Build history of the part. All positions in model axes, mm. A direction names the side the tool comes from. Coordinates: 2 decimals unless noted, no trailing zeros. Write each loop counter-clockwise with the first axis right and the second up, starting at its lowest first coordinate (ties: lowest second). Pieces come first, ordered by that corner, then holes. Notation, with made-up numbers: M 85.25,16 L 112.25,16 A14 ccw 112.25,33 Z; hole C -5,-4.5 d8. An arc over 180 degrees is marked long. Use CSV: the item, a comma, the result in double quotes. Start each with the question number.
```python
from build123d import *
from OCP.BRepFilletAPI import BRepFilletAPI_MakeChamfer

# Parameters (mm, degrees)
SKETCH_1_R          = 10
EXTRUDE_1_DEPTH     = 16.5
SKETCH_2_R          = 0.5
CUT_EXTRUDE_1_DEPTH = 6
SKETCH_3_R          = 8
CUT_EXTRUDE_2_DEPTH = 0.5
SKETCH_4_R          = 8.75
CUT_EXTRUDE_3_DEPTH = 0.8
SKETCH_5_R          = 0.8
EXTRUDE_2_DEPTH     = 4.85
CHAMFER_1_SIZE      = 2
CHAMFER_1_SIZE2     = 0.2
FILLET_1_R          = 0.4


with BuildPart() as part:
    # Эскиз1 → Бобышка-Вытянуть1 (new body)
    with BuildSketch(Plane.XY):
        Circle(SKETCH_1_R)
    extrude(amount=EXTRUDE_1_DEPTH)

    # Эскиз2 → Вырез-Вытянуть1 (cut)
    with BuildSketch(Plane.XY.offset(16.5)):
        Circle(SKETCH_2_R)
    extrude(amount=-CUT_EXTRUDE_1_DEPTH, mode=Mode.SUBTRACT)

    # Эскиз3 → Вырез-Вытянуть2 (cut)
    with BuildSketch(Plane.XY.offset(16.5)):
        Circle(SKETCH_3_R)
    extrude(amount=-CUT_EXTRUDE_2_DEPTH, mode=Mode.SUBTRACT)

    # Эскиз4 → Вырез-Вытянуть3 (cut)
    with BuildSketch(Plane(origin=(0, 0, 0), x_dir=(-1, 0, 0), z_dir=(0, 0, -1))):
        Circle(SKETCH_4_R)
    extrude(amount=-CUT_EXTRUDE_3_DEPTH, mode=Mode.SUBTRACT)

    # Эскиз5 → Бобышка-Вытянуть2 (add)
    with BuildSketch(Plane(origin=(0, 0, 0.8), x_dir=(-1, 0, 0), z_dir=(0, 0, -1))):
        with Locations((-4.7, 5)):
            Circle(SKETCH_5_R)
        with Locations(Location((4.7, 5, 0), (0, 0, 180))):
            Circle(SKETCH_5_R)
    extrude(amount=EXTRUDE_2_DEPTH)

    # Фаска1: one chamfer whose edges measure the first distance from different faces: ONE call of the kernel's chamfer builder (chamfer() names one face for all edges)
    chamfer_1_edges_1 = [part.edges().sort_by_distance(p)[0] for p in [
        (5.5, 5, -4.05),
    ]]
    chamfer_1_side_1 = [part.faces().sort_by_distance(p)[0] for p in [
        (5.5, 5, -1.625),
    ]]
    chamfer_1_edges_2 = [part.edges().sort_by_distance(p)[0] for p in [
        (-5.5, 5, -4.05),
    ]]
    chamfer_1_side_2 = [part.faces().sort_by_distance(p)[0] for p in [
        (-5.5, 5, -1.625),
    ]]
    chamfer_1 = BRepFilletAPI_MakeChamfer(part.part.solid().wrapped)
    for e in chamfer_1_edges_1:
        chamfer_1.Add(CHAMFER_1_SIZE, CHAMFER_1_SIZE2, e.wrapped, chamfer_1_side_1[0].wrapped)  # the first distance lies on this face
    for e in chamfer_1_edges_2:
        chamfer_1.Add(CHAMFER_1_SIZE, CHAMFER_1_SIZE2, e.wrapped, chamfer_1_side_2[0].wrapped)  # the first distance lies on this face
    add(Compound.cast(chamfer_1.Shape()), mode=Mode.REPLACE)

    # Скругление1
    fillet_1_edges = [part.edges().sort_by_distance(p)[0] for p in [
        (-8, 0, 16.5),
        (-10, 0, 0),
        (8.75, 0, 0),
        (-10, 0, 16.5),
    ]]
    fillet(fillet_1_edges, radius=FILLET_1_R)


solid = part.part
```
1. Slice it at A-A (z = 13.25). List the corners of the cut face in (x, y).
2. Drill centre lines: line 1 along Y through (x, z) = (0, 0.55); line 2 along Y through (x, z) = (0, 13.8); line 3 along Z through (x, y) = (2, 2). Where is each one in solid material? Low to high. Write a range as from..to.
3. Flat gauge pins, fed straight in: pin 1 (1.5 mm diameter, centred on x = -2.5, y = 2, fed in from +Z); pin 2 (2 mm diameter, centred on x = 7, y = 1.5, fed in from +Z); pin 3 (9 mm diameter, centred on x = 0, y = -1, fed in from -Z). Where does each tip first touch, or does it go through?
4. Slice it at C-C (z = -1). List the corners of the cut face in (x, y).
5. Pull direction X, two halves, no side cores. Call faces 1 (the cylindrical face through (5.33, 4.51, -0.61)), 2 (the cylindrical face through (-2.17, -9.76, 8.14)), 3 (the flat face through (-5, 5, -4.05)): pulls with the +X half, pulls with the -X half, needs draft (parallel to the pull), parting line crosses it, or undercut.
6. 3-axis set-ups, long thin cutter, end or side, ignore diameter. For faces 4 (the cylindrical face through (-4.87, 5.78, -0.61)), 5 (the flat face through (0, 0, 10.5)), 6 (the flat face through (5, 5, -4.05)): which of +Z, -Z, +X, -X, +Y, -Y reach the whole face in a straight line?
7. Slice it at B-B (y = 0). List the corners of the cut face in (x, z).
8. Slice it at D-D (z = 7.75). List the corners of the cut face in (x, y), and give its area (3 significant figures).
Established:
1,outline,"C 0,0 d20; hole C 0,0 d1"
2,line 1,"y = -10..-8.75, 8.75..10"
2,line 2,"y = -10..-0.5, 0.5..10"
2,line 3,"z = 0.8..16"
3,pin 1,"stops at z = 16"
3,pin 2,"stops at z = 16.42"
3,pin 3,"stops at z = 0.8"
4,outline,"C -4.7,5 d1.6; C 4.7,5 d1.6"
5,face 1,"undercut"
5,face 2,"parting line crosses it"
5,face 3,"needs draft"
6,face 4,"-Z"
6,face 5,"+Z"
6,face 6,"-Z, +X, -X, +Y, -Y"
7,outline,"M -10,0.4 A0.4 ccw -9.6,0 L -9.15,0 A0.4 ccw -8.75,0.4 L -8.75,0.8 L 8.75,0.8 L 8.75,0.4 A0.4 ccw 9.15,0 L 9.6,0 A0.4 ccw 10,0.4 L 10,16.1 A0.4 ccw 9.6,16.5 L 8.4,16.5 A0.4 ccw 8,16.1 L 8,16 L 0.5,16 L 0.5,10.5 L -0.5,10.5 L -0.5,16 L -8,16 L -8,16.1 A0.4 ccw -8.4,16.5 L -9.6,16.5 A0.4 ccw -10,16.1 Z"
8,outline,"C 0,0 d20"
8,area,"314 mm2"
